Check sheet for the modelled part. Datum: model origin and axes. Units: mm. Face numbers are marked on the shaded views. A direction names the side the tool comes from. Round coordinates to 2 decimals unless told otherwise and drop trailing zeros. Loops run counter-clockwise (first coordinate to the right, second up) from the corner with the lowest first, then second, coordinate; pieces in that order, holes last. Notation, with made-up numbers: M 6,72.25 L 61,72.25 A20 cw 61,110.25 Z; hole C 68,-8 d9. An arc over 180 degrees is marked long. One line per question, with ' | ' between items. Start each with the question number.
(1) Go/stop test with a flat-tipped pin: P1, Ø0.5, axis at x = 19.5, z = 0.5, coming from the -Y side (3 decimals). Record where the tip stops, or that it passes through.
(2) Section check B-B (x = 13). Record the boundary of the cut face in (y, z) (3 decimals), and give its area (3 significant figures).
(3) Thickness scan on probe 1 along Y at (x, z) = (17.5, 0.15) (3 decimals); probe 2 along X at (y, z) = (12.4, 0.5); probe 3 along X at (y, z) = (12.3, 0.85). Record the ranges inside material, lowest first. Write a range as [from, to].
(4) Tool access check on the marked faces 1, 2 and 3. Record the directions out of +Z, -Z, +X, -X, +Y, -Y that give a thin tool (end or side, any length) a straight path to the whole face; none if there is none.
(5) Section check C-C (y = 10.7). Record the boundary of the cut face in (x, z), and give its area (3 significant figures).
```python
from build123d import *

# Parameters (mm, degrees)
SHAPE_DEPTH = 1


with BuildPart() as part:
    # Sketch1 → Shape (new body)
    with BuildSketch(Plane.XY):
        with BuildLine():
            Line((17.307050808, 11.375), (21.274494937, 11.375))
            Line((21.274494937, 11.375), (23.074494937, 13.175))
            Line((23.074494937, 13.175), (8.75, 13.175))
            Line((8.75, 13.175), (8.75, 11.375))
            Line((8.75, 11.375), (13.842949192, 11.375))
            ThreePointArc((13.842949192, 11.375), (14.392949192, 11.227627944), (14.795577137, 10.825))
            ThreePointArc((14.795577137, 10.825), (15.575, 10.375), (16.354422863, 10.825))
            ThreePointArc((16.354422863, 10.825), (16.757050808, 11.227627944), (17.307050808, 11.375))
        make_face()
    extrude(amount=SHAPE_DEPTH)


solid = part.part
```
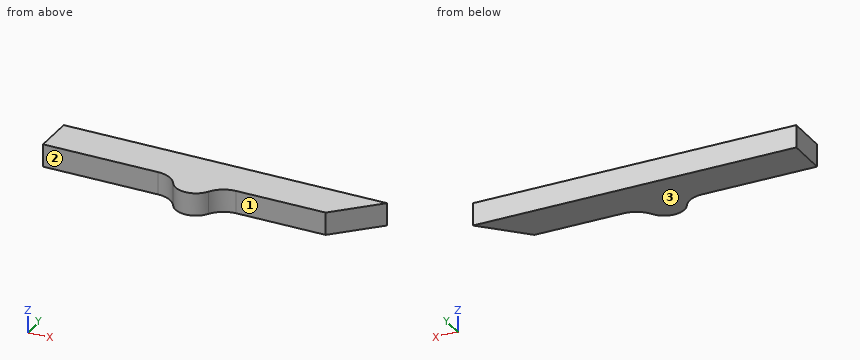
The answers:
1) P1: y = 11.375
2) outline: M 11.375,0 L 13.175,0 L 13.175,1 L 11.375,1 Z | area: 1.80 mm²
3) probe 1: [11.375, 13.175] | probe 2: [8.75, 22.3] | probe 3: [8.75, 22.2]
4) face 1: +Z, -Z, +X, -Y | face 2: +Z, -Z, -X, -Y | face 3: -Z, +X, -X, +Y, -Y
5) outline: M 14.88,0 L 16.27,0 L 16.27,1 L 14.88,1 Z | area: 1.38 mm²
